The listing builds one solid part. Answer for the finished solid, in the listing's coordinates (mm). A direction names the side the tool comes from. Give positions to 0.01 mm unless a question says otherwise; leave off trailing zeros. Order: outer loops, then holes, each group sorted by start corner. A loop starts at its lowest first (then second) coordinate and runs counter-clockwise, first axis right, second up. Notation, with made-up numbers: (5, 18.5) - (53, 18.5) arc R30 cw to (53, 45.5) - close; hole circle Ø2 at (73.25, 60.5). An arc over 180 degrees is marked (long way). Answer in a Markdown table with one row per item.
from build123d import *

# Parameters (mm, degrees)
SKETCH001_W    = 139
SKETCH001_H    = 84
PAD_DEPTH      = 25
THICKNESS_T    = 2
SKETCH002_R    = 5.947053
SKETCH002_R_2  = 6.391543
SKETCH002_R_3  = 7.479707
SKETCH002_R_4  = 6.690044
SKETCH002_R_5  = 7.551468
SKETCH002_R_6  = 6.341994
SKETCH002_R_7  = 8.509486
SKETCH002_R_8  = 9.409582
SKETCH002_R_9  = 8.069876
SKETCH002_R_10 = 7.030828
SKETCH002_R_11 = 5.146618
SKETCH002_R_12 = 6.982672
SKETCH002_R_13 = 7.752117
SKETCH002_R_14 = 10.787845
SKETCH002_R_15 = 5.65876
SKETCH002_R_16 = 3.93116
SKETCH002_R_17 = 3.377122
SKETCH002_R_18 = 5.622868
SKETCH002_R_19 = 3.905324
SKETCH002_R_20 = 4.228889
SKETCH002_R_21 = 3.528588
SKETCH002_R_22 = 3.16034
SKETCH002_R_23 = 6.106178
SKETCH002_R_24 = 4.85306
POCKET_DEPTH   = 5


with BuildPart() as part:
    # Sketch001 → Pad (new body)
    with BuildSketch(Plane.XY):
        with Locations((-29.136072, -13.413577)):
            Rectangle(SKETCH001_W, SKETCH001_H)
    extrude(amount=PAD_DEPTH)

    # Thickness
    thickness_openings = [part.faces().sort_by_distance(p)[0] for p in [
        (-98.636072, -13.413577, 12.5),
    ]]
    offset(amount=THICKNESS_T, openings=thickness_openings)

    # Sketch002 (on Face14 of Thickness) → Pocket (cut)
    with BuildSketch(Plane.XY.offset(27)):
        with Locations((-82.334571, 15.216334)):
            Circle(SKETCH002_R)
        with Locations((-61.021297, 18.021215)):
            Circle(SKETCH002_R_2)
        with Locations((-57.73288, -7.189993)):
            Circle(SKETCH002_R_3)
        with Locations((-86.232513, -9.656311)):
            Circle(SKETCH002_R_4)
        with Locations((-68.946266, -24.274019)):
            Circle(SKETCH002_R_5)
        with Locations((-82.723099, -44.663734)):
            Circle(SKETCH002_R_6)
        with Locations((-47.27071, -36.765015)):
            Circle(SKETCH002_R_7)
        with Locations((-30.922209, -11.599332)):
            Circle(SKETCH002_R_8)
        with Locations((-37.351395, 18.526012)):
            Circle(SKETCH002_R_9)
        with Locations((-17.329054, -28.866299)):
            Circle(SKETCH002_R_10)
        with Locations((-20.819183, -43.377895)):
            Circle(SKETCH002_R_11)
        with Locations((-12.920469, 15.403262)):
            Circle(SKETCH002_R_12)
        with Locations((9.489837, 16.872791)):
            Circle(SKETCH002_R_13)
        with Locations((-4.286991, -7.558129)):
            Circle(SKETCH002_R_14)
        with Locations((0, -29.968445)):
            Circle(SKETCH002_R_15)
        with Locations((-44.858665, 4.777251)):
            Circle(SKETCH002_R_16)
        with Locations((-74.249245, 5.328322)):
            Circle(SKETCH002_R_17)
        with Locations((-64.697304, -45.003048)):
            Circle(SKETCH002_R_18)
        with Locations((-36.225178, -46.839958)):
            Circle(SKETCH002_R_19)
        with Locations((-33.469814, -28.103462)):
            Circle(SKETCH002_R_20)
        with Locations((-49.450947, -18.551527)):
            Circle(SKETCH002_R_21)
        with Locations((-28.142773, 7.716309)):
            Circle(SKETCH002_R_22)
        with Locations((-5.732456, -45.003048)):
            Circle(SKETCH002_R_23)
        with Locations((-89.679298, -27.368698)):
            Circle(SKETCH002_R_24)
    extrude(amount=-POCKET_DEPTH, mode=Mode.SUBTRACT)


solid = part.part
Item 1: Consider line 1 (Z direction, x = 33, y = 4.5); line 2 (Y direction, x = -10, z = 2.5); line 3 (X direction, y = -7.5, z = 17.5). Determine where each line is inside the solid, lowest interval first.
Answer block:
| item | result |
|---|---|
| line 1 | -2 to 0, 25 to 27 |
| line 2 | -57.41 to -55.41, 28.59 to 30.59 |
| line 3 | 40.36 to 42.36 |
Item 2: Find section C-C on x = 12. Write down the section's boundary in (y, z), then the cut area to 3 significant figures.
Answer block:
| item | result |
|---|---|
| outline | (-57.41, 0) arc R2 ccw to (-55.41, -2) - (28.59, -2) arc R2 ccw to (30.59, 0) - (30.59, 25) arc R2 ccw to (28.59, 27) - (24.21, 27) - (24.21, 25) - (28.59, 25) - (28.59, 0) - (-55.41, 0) - (-55.41, 25) - (9.54, 25) - (9.54, 27) - (-55.41, 27) arc R2 ccw to (-57.41, 25) - close |
| area | 419 mm² |
Item 3: Find section B-B on z = 5. Write down the section's boundary in (x, y).
Answer block:
| item | result |
|---|---|
| outline | (-98.64, -57.41) - (40.36, -57.41) arc R2 ccw to (42.36, -55.41) - (42.36, 28.59) arc R2 ccw to (40.36, 30.59) - (-98.64, 30.59) - (-98.64, 28.59) - (40.36, 28.59) - (40.36, -55.41) - (-98.64, -55.41) - close |
Item 4: Determine the mould class of faces 3 (the face through (-84.098, -50.855, 26.014)), 4 (the face through (-30, -22, 27)) for opening direction Y: pulls with the +Y half, pulls with the -Y half, needs draft (parallel to the pull), parting line crosses it, or undercut.
Answer block:
| item | result |
|---|---|
| face 3 | undercut |
| face 4 | needs draft |
Item 5: Find section A-A on y = -13. Write down the section's boundary in (x, z), then the cut area to 3 significant figures.
Answer block:
| item | result |
|---|---|
| outline | (-98.64, -2) - (40.36, -2) arc R2 ccw to (42.36, 0) - (42.36, 25) arc R2 ccw to (40.36, 27) - (5.03, 27) - (5.03, 25) - (40.36, 25) - (40.36, 0) - (-98.64, 0) - close; (-98.64, 25) - (-92.03, 25) - (-92.03, 27) - (-98.64, 27) - close; (-80.44, 25) - (-62.44, 25) - (-62.44, 27) - (-80.44, 27) - close; (-53.02, 25) - (-40.23, 25) - (-40.23, 27) - (-53.02, 27) - close; (-21.62, 25) - (-13.6, 25) - (-13.6, 27) - (-21.62, 27) - close |
| area | 496 mm² |
Item 6: Each of these flat-tipped pins is pushed along its axis until it touches: P1, Ø1.5, axis at y = -35.5, z = 14, coming from the -X side; P2, Ø4, axis at x = -74.25, y = 5.33, coming from the +Z side. Where does it stop, or does it pass through?
Answer block:
| item | result |
|---|---|
| P1 | x = 40.36 |
| P2 | z = 0 |
Item 7: Which of the six approach directions +Z, -Z, +X, -X, +Y, -Y give full straight-line access (tool end or side, diameter ignored) to faces 1 (the face through (-71.028, 6.343, 26.014)), 2 (the face through (-30, -22, 25))?
Answer block:
| item | result |
|---|---|
| face 1 | +Z |
| face 2 | -X |
